Build history of the part. All positions in model axes, mm. A direction names the side the tool comes from. Round coordinates to 2 decimals unless told otherwise and drop trailing zeros. Loops run counter-clockwise (first coordinate to the right, second up) from the corner with the lowest first, then second, coordinate; pieces in that order, holes last. Notation, with made-up numbers: (-14, -14.75) -> (19, -14.75) arc R31 ccw to (19, 9.25) -> close; hole circle Ø6 at (27.25, 66). An arc over 180 degrees is marked (long way). Put each result on its own line as item: value. Start each with the question number.
```python
from build123d import *

# Parameters (mm, degrees)
SKETCH_1_W      = 194
SKETCH_1_H      = 90
EXTRUDE_1_DEPTH = 3


with BuildPart() as part:
    # 草圖1 → 填料-伸長1 (new body)
    with BuildSketch(Plane.XY):
        with Locations((-1.5, 0.009137056)):
            Rectangle(SKETCH_1_W, SKETCH_1_H)
        Polygon((50.5, -20.847715736), (50.5, -0.847715736), (90.5, 4.009137056), (90.5, -15.990862944), align=None, mode=Mode.SUBTRACT)
        Polygon((2.5, -26.695431472), (2.5, -4.695431472), (42.5, 0.177664975), (42.5, -21.822335025), align=None, mode=Mode.SUBTRACT)
        Polygon((-45.5, -32.543147208), (-45.5, -6.543147208), (-5.5, -1.670050761), (-5.5, -27.670050761), align=None, mode=Mode.SUBTRACT)
        Polygon((-93.5, -38.390862944), (-93.5, -10.390862944), (-53.5, -5.517766497), (-53.5, -33.517766497), align=None, mode=Mode.SUBTRACT)
    extrude(amount=EXTRUDE_1_DEPTH)


solid = part.part
```
Item 1: 3-axis set-ups, long thin cutter, end or side, ignore diameter. For faces 3 (the face through (-3, 1, 3)), 4 (the face through (70.22, 1.547, 1.479)): which of +Z, -Z, +X, -X, +Y, -Y reach the whole face in a straight line?
Item 2: Pull direction Y, two halves, no side cores. Call faces 1 (the face through (-3, 1, 0)), 2 (the face through (-25.78, -4.14, 1.48)): +Y half, -Y half, draft (parallel to the pull), parting line (faces both ways), or undercut.
Item 3: Cut at A-A on z = 0.5. Write the cut outline in (x, y), then the cut area to 3 significant figures.
Item 4: Cut at B-B on x = -11.5. Write the cut outline in (y, z).
Item 5: Wall check: line 1 (X direction, y = -13.5, z = 1.95); line 2 (Y direction, x = 20, z = 1.6); line 3 (Y direction, x = 37, z = 2.45). Give the ranges that are in metal, low to high. Write a range as from..to.
Item 6: Cut at C-C on x = 38.5. Write the cut outline in (y, z).
Ans:
1. face 3: +Z, +X, -X, +Y, -Y
1. face 4: +Z, -Z
2. face 1: draft
2. face 2: undercut
3. outline: (-98.5, -44.99) -> (95.5, -44.99) -> (95.5, 45.01) -> (-98.5, 45.01) -> close; hole (-93.5, -38.39) -> (-53.5, -33.52) -> (-53.5, -5.52) -> (-93.5, -10.39) -> close; hole (-45.5, -32.54) -> (-5.5, -27.67) -> (-5.5, -1.67) -> (-45.5, -6.54) -> close; hole (2.5, -26.7) -> (42.5, -21.82) -> (42.5, 0.18) -> (2.5, -4.7) -> close; hole (50.5, -20.85) -> (90.5, -15.99) -> (90.5, 4.01) -> (50.5, -0.85) -> close
3. area: 13,600 mm2
4. outline: (-44.99, 0) -> (-28.4, 0) -> (-28.4, 3) -> (-44.99, 3) -> close; (-2.4, 0) -> (45.01, 0) -> (45.01, 3) -> (-2.4, 3) -> close
5. line 1: x = -98.5..-93.5, -53.5..-45.5, -5.5..2.5, 42.5..50.5, 90.5..95.5
5. line 2: y = -44.99..-24.56, -2.56..45.01
5. line 3: y = -44.99..-22.49, -0.49..45.01
6. outline: (-44.99, 0) -> (-22.31, 0) -> (-22.31, 3) -> (-44.99, 3) -> close; (-0.31, 0) -> (45.01, 0) -> (45.01, 3) -> (-0.31, 3) -> close
